Work out the finished part from the listing and answer in its coordinate system (mm). A direction names the side the tool comes from. Give positions to 0.01 mm unless a question says otherwise; leave off trailing zeros. Write each loop counter-clockwise with the first axis right and the second up, starting at its lowest first coordinate (ties: lowest second). Pieces come first, ordered by that corner, then holes.
1) Straight lines are drawn through the part: probe 1 along Z at (x, y) = (123, 23); probe 2 along Z at (x, y) = (78, 75). For each, find the intervals that lie inside material, in ascending order.
2) Find section A-A (x = 84). Determine the outline of the cut face in (y, z).
3) Find section B-B (y = 37). Determine the outline of the cut face in (x, z), plus the area to 3 significant figures.
4) Given pin 1 Ø12 at (x, y) = (70.5, 54) entering from +Z; pin 2 Ø12 at (y, z) = (83, 152) entering from +X, each flat-ended and moving along its own axis, determine where each tip first touches the part or whether it passes through.
5) A tool of negligible diameter and unlimited length cuts with its end or side. For faces 1 (the face through (66, 5, 273)), 2 (the face through (125, 1, 141)), 3 (the face through (0, 9, 162)), 4 (the face through (5, 10, 136)), 5 (the face through (130, 91, 163)), from which of +Z, -Z, +X, -X, +Y, -Y can it reach the whole face along a straight path? Write none if from no direction.
6) Find section C-C (z = 154). Count the separate pieces of the cut face and the enclosed holes in it, plus the area to 3 significant figures.
7) Determine the mould class of faces 6 (the face through (120, 49, 278)), 7 (the face through (125, 10, 136)) for opening direction Z: pulls with the +Z half, pulls with the -Z half, needs draft (parallel to the pull), parting line crosses it, or undercut.
```python
from build123d import *

# Parameters (mm, degrees)
SKETCH1_W           = 130
SKETCH1_H           = 100
BOSS_EXTRUDE1_DEPTH = 3
SKETCH2_W           = 10
SKETCH2_H           = 10
SKETCH2_W_2         = 7
SKETCH2_H_2         = 7
BOSS_EXTRUDE2_DEPTH = 280
SKETCH3_W           = 10
SKETCH3_H           = 10
SKETCH3_W_2         = 7
SKETCH3_H_2         = 7
BOSS_EXTRUDE3_DEPTH = 112
SKETCH4_W           = 10
SKETCH4_H           = 10
SKETCH4_W_2         = 7
SKETCH4_H_2         = 7
BOSS_EXTRUDE4_DEPTH = 112
SKETCH5_W           = 10
SKETCH5_H           = 10
SKETCH5_W_2         = 7
SKETCH5_H_2         = 7
BOSS_EXTRUDE5_DEPTH = 82
SKETCH6_W           = 10
SKETCH6_H           = 10
SKETCH6_W_2         = 7
SKETCH6_H_2         = 7
BOSS_EXTRUDE6_DEPTH = 82
SKETCH7_W           = 7
SKETCH7_H           = 7
SKETCH7_W_2         = 6
BOSS_EXTRUDE7_DEPTH = 0.1


with BuildPart() as part:
    # Sketch1 → Boss-Extrude1 (new body)
    with BuildSketch(Plane.XY):
        with Locations((65, 50)):
            Rectangle(SKETCH1_W, SKETCH1_H)
    extrude(amount=BOSS_EXTRUDE1_DEPTH)

    # Sketch2 → Boss-Extrude2 (add)
    # profile 1 of 4: a face of its own
    with BuildSketch(Plane.XY.offset(3)):
        with Locations((125, 95)):
            Rectangle(SKETCH2_W, SKETCH2_H)
        with Locations((125.5, 95.5)):
            Rectangle(SKETCH2_W_2, SKETCH2_H_2, mode=Mode.SUBTRACT)
    # profile 2 of 4: a face of its own
    with BuildSketch(Plane.XY.offset(3)):
        with Locations((125, 5)):
            Rectangle(SKETCH2_W, SKETCH2_H)
        with Locations((125.5, 4.5)):
            Rectangle(SKETCH2_W_2, SKETCH2_H_2, mode=Mode.SUBTRACT)
    # profile 3 of 4: a face of its own
    with BuildSketch(Plane.XY.offset(3)):
        with Locations((5, 5)):
            Rectangle(SKETCH2_W, SKETCH2_H)
        with Locations((5.5, 4.5)):
            Rectangle(SKETCH2_W_2, SKETCH2_H_2, mode=Mode.SUBTRACT)
    # profile 4 of 4: a face of its own
    with BuildSketch(Plane.XY.offset(3)):
        with Locations((5, 95)):
            Rectangle(SKETCH2_W, SKETCH2_H)
        with Locations((4.5, 95.5)):
            Rectangle(SKETCH2_W_2, SKETCH2_H_2, mode=Mode.SUBTRACT)
    extrude(amount=BOSS_EXTRUDE2_DEPTH)

    # Sketch3 → Boss-Extrude3 (add)
    with BuildSketch(Plane.ZY.offset(-120)):
        with Locations((278, 95)):
            Rectangle(SKETCH3_W, SKETCH3_H)
        with Locations((278, 95)):
            Rectangle(SKETCH3_W_2, SKETCH3_H_2, mode=Mode.SUBTRACT)
    extrude(amount=BOSS_EXTRUDE3_DEPTH)

    # Sketch4 → Boss-Extrude4 (add)
    with BuildSketch(Plane.ZY.offset(-120)):
        with Locations((278, 5)):
            Rectangle(SKETCH4_W, SKETCH4_H)
        with Locations((278, 5)):
            Rectangle(SKETCH4_W_2, SKETCH4_H_2, mode=Mode.SUBTRACT)
    extrude(amount=BOSS_EXTRUDE4_DEPTH)

    # Sketch5 → Boss-Extrude5 (add)
    with BuildSketch(Plane(origin=(0, 10, 0), x_dir=(1, 0, 0), z_dir=(0, 1, 0))):
        with Locations((125, -278)):
            Rectangle(SKETCH5_W, SKETCH5_H)
        with Locations((125, -278)):
            Rectangle(SKETCH5_W_2, SKETCH5_H_2, mode=Mode.SUBTRACT)
    extrude(amount=BOSS_EXTRUDE5_DEPTH)

    # Sketch6 → Boss-Extrude6 (add)
    with BuildSketch(Plane.XZ.offset(-90)):
        with Locations((5, 278)):
            Rectangle(SKETCH6_W, SKETCH6_H)
        with Locations((5, 278)):
            Rectangle(SKETCH6_W_2, SKETCH6_H_2, mode=Mode.SUBTRACT)
    extrude(amount=BOSS_EXTRUDE6_DEPTH)

    # Sketch7 → Boss-Extrude7 (add)
    with BuildSketch(Plane.XY.offset(283)):
        with Locations((4.5, 95.5)):
            Rectangle(SKETCH7_W, SKETCH7_H)
        with Locations((125.5, 95.5)):
            Rectangle(SKETCH7_W, SKETCH7_H)
        with Locations((125.5, 4.5)):
            Rectangle(SKETCH7_W, SKETCH7_H)
        with Locations((5, 4.5)):
            Rectangle(SKETCH7_W_2, SKETCH7_H)
    extrude(amount=-BOSS_EXTRUDE7_DEPTH)


solid = part.part
```
Results:
1. probe 1: z = 0 to 3, 273 to 274.5, 281.5 to 283
1. probe 2: z = 0 to 3
2. outline: (0, 0) - (100, 0) - (100, 3) - (0, 3) - close; (0, 273) - (10, 273) - (10, 283) - (0, 283) - close; (90, 273) - (100, 273) - (100, 283) - (90, 283) - close; hole (1.5, 274.5) - (8.5, 274.5) - (8.5, 281.5) - (1.5, 281.5) - close; hole (91.5, 274.5) - (98.5, 274.5) - (98.5, 281.5) - (91.5, 281.5) - close
3. outline: (0, 0) - (130, 0) - (130, 3) - (0, 3) - close; (0, 273) - (10, 273) - (10, 283) - (0, 283) - close; (120, 273) - (130, 273) - (130, 283) - (120, 283) - close; hole (1.5, 274.5) - (8.5, 274.5) - (8.5, 281.5) - (1.5, 281.5) - close; hole (121.5, 274.5) - (128.5, 274.5) - (128.5, 281.5) - (121.5, 281.5) - close
3. area: 492 mm2
4. pin 1: stops at z = 3
4. pin 2: passes through
5. face 1: +Y, -Y
5. face 2: none
5. face 3: +Z, -Z, -X, +Y, -Y
5. face 4: +X, -X
5. face 5: +Z, -Z, +X, +Y, -Y
6. separate pieces: 4
6. enclosed holes: 4
6. area: 204 mm2
7. face 6: needs draft
7. face 7: undercut
